Autodesk Inventor part; units mm, degrees
ref_plane "YZ Plane" through (0, 0, 0) normal (1, 0, 0) x (0, 1, 0)
ref_plane "XZ Plane" through (0, 0, 0) normal (0, 1, 0) x (-1, 0, 0)
ref_plane "XY Plane" through (0, 0, 0) normal (0, 0, 1) x (1, 0, 0)
sketch "Skizze1" plane through (0, 0, 0) normal (0, 0, 1) x (1, 0, 0)
  line L0 (-2.15, 4.15) -> (2.15, 4.15)
  line L1 (4.15, 2.15) -> (4.15, -2.15)
  line L2 (2.15, -4.15) -> (-2.15, -4.15)
  line L3 (-4.15, -2.15) -> (-4.15, 2.15)
  arc A0 (-2.15, 4.15) -> (-4.15, 2.15) centre (-2.15, 2.15) ccw
  arc A1 (4.15, 2.15) -> (2.15, 4.15) centre (2.15, 2.15) ccw
  arc A2 (2.15, -4.15) -> (4.15, -2.15) centre (2.15, -2.15) ccw
  arc A3 (-4.15, -2.15) -> (-2.15, -4.15) centre (-2.15, -2.15) ccw
  line L4 (-2.15, 2.15) -> (2.15, -2.15) construction
  line L5 (2.15, 2.15) -> (-2.15, -2.15) construction
  point P0 (0, 0)
  dimension "d0" = 2
  dimension "d1" = 8.3
extrude "Extrusion1" add sketch "Skizze1" along normal blind 3
sketch "Skizze2" plane through (0, 0, 3) normal (0, 0, 1) x (1, 0, 0)
  circle A0 centre (0, 0) radius 2.5
  circle A1 centre (0, 0) radius 3
  dimension "d4" = 5
  dimension "d22" = 6
extrude "Extrusion2" add sketch "Skizze2" along normal blind 12 contours A0
sketch "Skizze3" plane through (0, 0, 15) normal (0, 0, 1) x (1, 0, 0)
  point P0 (0, 0)
  point P1 (0, 0)
hole "Bohrung1" at (0, 0, 15) direction (0, 0, -1) diameter 3 end through all
chamfer "Fase1" distance 0.5 angle 45 1 edges at (-2.5, 0, 15)
thread "Gewinde2"
extrude "Extrusion3" add sketch "Skizze2" along normal blind 6.2
sketch "Skizze4" plane through (0, 0, 0) normal (0, 0, -1) x (-1, 0, 0)
  point P0 (0, 0)
  point P1 (0, 0)
hole "Bohrung2" [suppressed]
chamfer "Fasen2" distance 0.1 angle 45 2 edges at (-3, 0, 9.2) (0, 1.5, 0)
chamfer "Fasen3" [suppressed]
properties part number "Radadapter" material "Aluminium 6061"
Model file for the job. Use its own axes, mm. A direction names the side the tool comes from. Round coordinates to 2 decimals unless told otherwise and drop trailing zeros. Order: outer loops, then holes, each group sorted by start corner. A loop starts at its lowest first (then second) coordinate and runs counter-clockwise, first axis right, second up. Notation, with made-up numbers: M 26.5,30 L 77.5,30 A31 ccw 77.5,66 Z; hole C -26,19 d8. An arc over 180 degrees is marked long. Write each question's results on one line, items separated by ' | '. Start each with the question number.
(1) Saw through at D-D, the plane x = 3.75. Give the cut face in (y, z), then the cut area to 3 significant figures.
(2) Saw through at C-C, the plane z = 12.25. Give the cut face in (x, y), then the cut area to 3 significant figures.
(3) Which spindle directions (+Z, -Z, +X, -X, +Y, -Y) get a long thin tool onto all of the face, cutting with end or side? Do faces 4 (the face through (-0.54, 2.44, 11.81)), 5 (the face through (0, -4.15, 1)). Say none if no direction does.
(4) Saw through at A-A, the plane y = 0. Give the cut face in (x, z), then the cut area to 3 significant figures.
(5) Drop a flat-ended pin along its axis: pin 1 (1.7 mm diameter, centred on x = 0, y = 0, fed in from +Z). Give the stop position or say it passes through.
(6) Two-plate mould, pull along X, no slides. Class faces 1 (the face through (3.55, 3.58, 1.48)), 2 (the face through (-3.58, 3.55, 1.48)), 3 (the face through (-0.07, 1.5, 7.45)): pulls with the +X half, pulls with the -X half, needs draft (parallel to the pull), parting line crosses it, or undercut.
(7) Probe probe 1 along Y at (x, z) = (0, 7.25); probe 2 along Y at (x, z) = (0, 11); probe 3 along Z at (x, y) = (3.5, 2.25). List the from-to ranges inside material, lowest first. Write a range as from..to.
Established:
1) outline: M -3.35,0 L 3.35,0 L 3.35,3 L -3.35,3 Z | area: 20.1 mm^2
2) outline: C 0,0 d5; hole C 0,0 d3 | area: 12.6 mm^2
3) face 4: +Z | face 5: +Z, -Z, +X, -X, -Y
4) outline: M -4.15,0 L -1.6,0 L -1.5,0.1 L -1.5,15 L -2,15 L -2.5,14.5 L -2.5,9.2 L -2.9,9.2 L -3,9.1 L -3,3 L -4.15,3 Z; M 1.5,0.1 L 1.6,0 L 4.15,0 L 4.15,3 L 3,3 L 3,9.1 L 2.9,9.2 L 2.5,9.2 L 2.5,14.5 L 2,15 L 1.5,15 Z | area: 45.8 mm^2
5) pin 1: passes through
6) face 1: pulls with the +X half | face 2: pulls with the -X half | face 3: undercut
7) probe 1: y = -3..-1.5, 1.5..3 | probe 2: y = -2.5..-1.5, 1.5..2.5 | probe 3: z = 0..3
